```python
from build123d import *

# Parameters (mm, degrees)
SKETCH_2_R          = 2
EXTRUDE_1_DEPTH     = 6
EXTRUDE_START       = -1.8
EXTRUDE_2_DEPTH     = 1.8
SKETCH_6_W          = 30
SKETCH_6_H          = 30
EXTRUDE_3_DEPTH     = 10
SKETCH_7_W          = 5
SKETCH_7_H          = 20
CUT_EXTRUDE_1_DEPTH = 37.936034472
FILLET_1_R          = 1


# Read off the part's stored shape, not the designer's step: the extrude step
with BuildPart() as part:
    # Sketch 2 → Extrude 1 (new body)
    with BuildSketch(Plane(origin=(0, 0, 0), x_dir=(0, 0, -1), z_dir=(1, 0, 0))):
        Circle(SKETCH_2_R)
    extrude(amount=-EXTRUDE_1_DEPTH)

    # Extrude 2 outline → Extrude 2 (add)
    with BuildSketch(Plane(origin=(-2, 0, 0), x_dir=(0, 0, -1), z_dir=(1, 0, 0)).offset(EXTRUDE_START)):
        with BuildLine():
            Line((15, 16.573624844), (12.700200279, 18.5))
            Line((12.700200279, 18.5), (-0.300448261, 1.977303933))
            ThreePointArc((-0.300448261, 1.977303933), (1.284250104, 1.533199814), (1.99935146, 0.050928777))
            Line((1.99935146, 0.050928777), (15, 16.573624844))
        make_face()
        with BuildLine():
            ThreePointArc((0.300448261, -1.977303933), (-1.284250104, -1.533199814), (-1.99935146, -0.050928777))
            Line((-1.99935146, -0.050928777), (-15, -17.159500316))
            Line((-15, -17.159500316), (-12.700200279, -19.085875472))
            Line((-12.700200279, -19.085875472), (0.300448261, -1.977303933))
        make_face()
    extrude(amount=EXTRUDE_2_DEPTH)

    # Sketch 6 → Extrude 3 (add)
    with BuildSketch(Plane(origin=(0, 0, 0), x_dir=(0, 0, -1), z_dir=(1, 0, 0))):
        Rectangle(SKETCH_6_W, SKETCH_6_H)
    extrude(amount=EXTRUDE_3_DEPTH)

    # Sketch 7 → Cut-Extrude 1 (cut, through all)
    with BuildSketch(Plane.XY.offset(15)):
        with Locations((5, 0)):
            Rectangle(SKETCH_7_W, SKETCH_7_H)
    extrude(amount=-CUT_EXTRUDE_1_DEPTH, mode=Mode.SUBTRACT)

    # Fillet 1
    fillet_1_edges = [part.edges().sort_by_distance(p)[0] for p in [
        (5, 15, 15),
        (5, -15, 15),
        (5, -15, -15),
        (5, 15, -15),
        (10, 0, 15),
        (10, -15, 0),
        (10, 0, -15),
        (10, 15, 0),
    ]]
    fillet(fillet_1_edges, radius=FILLET_1_R)


solid = part.part
```
For this review, take the finished solid that the model builds, in its own axes (mm). A direction names the side the tool comes from. Round coordinates to 2 decimals unless told otherwise and drop trailing zeros. Write each loop counter-clockwise with the first axis right and the second up, starting at its lowest first coordinate (ties: lowest second). Pieces come first, ordered by that corner, then holes.
1) For line 1 along X through (y, z) = (5, -5.25); line 2 along Y through (x, z) = (6, 12.5); line 3 along X through (y, z) = (7.5, -12.25), list the stretches that pass through material, from the lowest coordinate up.
Answer below:
line 1: x = -3.8 to -2, 0 to 2.5, 7.5 to 10
line 2: y = -15 to -10, 10 to 15
line 3: x = 0 to 2.5, 7.5 to 10
2) Take a section at D-D on z = -1.5. Give the boundary of the cut face in (x, y).
Answer below:
outline: (-6, -1.32) - (0, -1.32) - (0, -15) - (9, -15) arc R1 ccw to (10, -14) - (10, 14) arc R1 ccw to (9, 15) - (0, 15) - (0, 1.32) - (-2, 1.32) - (-2, 4.27) - (-3.8, 4.27) - (-3.8, 1.32) - (-6, 1.32) - close; hole (2.5, -10) - (7.5, -10) - (7.5, 10) - (2.5, 10) - close
3) Insertion check: pin 1 Ø3 at (x, y) = (-2.5, 11.5) entering from +Z; pin 2 Ø8 at (x, z) = (-1.5, -7.5) entering from -Y; pin 3 Ø7 at (x, z) = (4, 0.5) entering from +Y. Each pin has a flat end and moves straight along its axis. Give the tip position at first contact, or say it passes through.
Answer below:
pin 1: stops at z = -6.01
pin 2: stops at y = -15
pin 3: stops at y = 15
4) Take a section at B-B on z = -10. Give the boundary of the cut face in (x, y).
Answer below:
outline: (-3.8, 10.22) - (-2, 10.22) - (-2, 15.07) - (-3.8, 15.07) - close; (0, -15) - (9, -15) arc R1 ccw to (10, -14) - (10, 14) arc R1 ccw to (9, 15) - (0, 15) - close; hole (2.5, -10) - (7.5, -10) - (7.5, 10) - (2.5, 10) - close
5) Mouldability with a two-part tool opening along X and no side actions: class faces 4 (the face through (7.5, 0, 0)), 5 (the face through (-2.913, -18.109, 13.866)), 6 (the face through (9.699, -14.715, -0.196)) as +X half, -X half, draft (parallel to the pull), parting line (faces both ways), or undercut.
Answer below:
face 4: undercut
face 5: draft
face 6: +X half
6) Take a section at C-C on y = 12.5. Give the boundary of the cut face in (x, z).
Answer below:
outline: (-3.8, -11.79) - (-2, -11.79) - (-2, -7.98) - (-3.8, -7.98) - close; (0, -15) - (9, -15) arc R1 ccw to (10, -14) - (10, 14) arc R1 ccw to (9, 15) - (0, 15) - close
7) Machinability: for faces 1 (the face through (-2.958, -1.774, -0.923)), 2 (the face through (-2.91, -10.65, 6.29)), 3 (the face through (2.5, 0, 0)), which of the approach directions +Z, -Z, +X, -X, +Y, -Y give a long, thin tool a straight path to every point of the face, cutting with its end or side? Answer none if there is none.
Answer below:
face 1: none
face 2: -Z, -X, -Y
face 3: +Z, -Z
8) Take a section at A-A on x = 7. Give the boundary of the cut face in (y, z), then the cut area to 3 significant figures.
Answer below:
outline: (-15, -14) arc R1 ccw to (-14, -15) - (-10, -15) - (-10, 15) - (-14, 15) arc R1 ccw to (-15, 14) - close; (10, -15) - (14, -15) arc R1 ccw to (15, -14) - (15, 14) arc R1 ccw to (14, 15) - (10, 15) - close
area: 299 mm2
